from build123d import *

# Parameters (mm, degrees)
F0_R     = 1.75
F0_R_2   = 7.5
F1_DEPTH = 3


with BuildPart() as f1:
    # F0 (on Top) → F1 (new body)
    with BuildSketch(Plane.XY):
        with BuildLine():
            Line((-37.25, -45), (37.25, -45))
            Line((37.25, -45), (37.25, 40))
            ThreePointArc((37.25, 40), (35.785534, 43.535534), (32.25, 45))
            Line((32.25, 45), (-32.25, 45))
            ThreePointArc((-32.25, 45), (-35.785534, 43.535534), (-37.25, 40))
            Line((-37.25, 40), (-37.25, -45))
        make_face()
        with Locations((-27.75, -37.05)):
            Circle(F0_R, mode=Mode.SUBTRACT)
        with Locations((-13, -30.9)):
            Circle(F0_R, mode=Mode.SUBTRACT)
        with Locations((-27.75, -13.25)):
            Circle(F0_R, mode=Mode.SUBTRACT)
        with Locations((-13, -19.4)):
            Circle(F0_R, mode=Mode.SUBTRACT)
        with Locations((0, -25.15)):
            Circle(F0_R_2, mode=Mode.SUBTRACT)
        with Locations((13, -30.9)):
            Circle(F0_R, mode=Mode.SUBTRACT)
        with Locations((27.75, -37.05)):
            Circle(F0_R, mode=Mode.SUBTRACT)
        with Locations((13, -19.4)):
            Circle(F0_R, mode=Mode.SUBTRACT)
        with Locations((27.75, -13.25)):
            Circle(F0_R, mode=Mode.SUBTRACT)
        with Locations((-28.25, 35.25)):
            Circle(F0_R, mode=Mode.SUBTRACT)
        with Locations((-15, 35.25)):
            Circle(F0_R, mode=Mode.SUBTRACT)
        with Locations((15, 35.25)):
            Circle(F0_R, mode=Mode.SUBTRACT)
        with Locations((28.25, 35.25)):
            Circle(F0_R, mode=Mode.SUBTRACT)
    extrude(amount=F1_DEPTH)


solid = f1.part
Here's how the part is built. I have some questions about the finished solid (model axes, mm). Round coordinates to 2 decimals unless told otherwise and drop trailing zeros. Write each loop counter-clockwise with the first axis right and the second up, starting at its lowest first coordinate (ties: lowest second). Pieces come first, ordered by that corner, then holes. Notation, with made-up numbers: (-38, 30.5) -> (3, 30.5) arc R31 ccw to (3, 58.5) -> close; hole circle Ø10 at (89.25, -7). An arc over 180 degrees is marked (long way). One line per item, written item: value.
1) I'm going to push a flat-ended pin straight in: pin 1 Ø6 at (x, y) = (-10, -11) entering from -Z. Where does the tip first touch, or does it pass through?
Filled sheet:
pin 1: stops at z = 0
2) Suppose I cut it at B-B on x = 0. List the corners of the cut face in (y, z) for me.
Filled sheet:
outline: (-45, 0) -> (-32.65, 0) -> (-32.65, 3) -> (-45, 3) -> close; (-17.65, 0) -> (45, 0) -> (45, 3) -> (-17.65, 3) -> close
3) We'd pull the mould along X, two halves only. Please class faces 1 (the face through (-12.19, -20.95, 1.48)), 2 (the face through (-1, -45, 1)), 3 (the face through (-35.75, 43.57, 1.48)): released by +X, released by -X, zero draft, split by the parting line, or undercut.
Filled sheet:
face 1: undercut
face 2: zero draft
face 3: released by -X
4) Suppose I cut it at D-D on z = 1.2. Give the number of separate pieces and of enclosed holes in the cut face, plus the area to 3 significant figures.
Filled sheet:
separate pieces: 1
enclosed holes: 13
area: 6,400 mm2
5) If I drill on line 1 (Y direction, x = -13, z = 2.4); line 2 (X direction, y = -13, z = 1.3); line 3 (Y direction, x = 0, z = 1), over which ranges is the centre line in solid material (lowest first)? Write a range as [from, to].
Filled sheet:
line 1: y = [-45, -32.65], [-29.15, -21.15], [-17.65, 45]
line 2: x = [-37.25, -29.48], [-26.02, 26.02], [29.48, 37.25]
line 3: y = [-45, -32.65], [-17.65, 45]
6) Suppose I cut it at A-A on y = -13.25. List the corners of the cut face in (x, z) for me.
Filled sheet:
outline: (-37.25, 0) -> (-29.5, 0) -> (-29.5, 3) -> (-37.25, 3) -> close; (-26, 0) -> (26, 0) -> (26, 3) -> (-26, 3) -> close; (29.5, 0) -> (37.25, 0) -> (37.25, 3) -> (29.5, 3) -> close
7) Suppose I cut it at C-C on y = -25.15. List the corners of the cut face in (x, z) for me.
Filled sheet:
outline: (-37.25, 0) -> (-7.5, 0) -> (-7.5, 3) -> (-37.25, 3) -> close; (7.5, 0) -> (37.25, 0) -> (37.25, 3) -> (7.5, 3) -> close
